For this review, take the finished solid that the model builds, in its own axes (mm). Coordinates: 2 decimals unless noted, no trailing zeros. Loops run counter-clockwise (first coordinate to the right, second up) from the corner with the lowest first, then second, coordinate; pieces in that order, holes last. Notation, with made-up numbers: M 6,50 L 64,50 A25 cw 64,77 Z; hole C 59,12 d5. An arc over 180 degrees is marked long. Put each result on its own line as item: value.
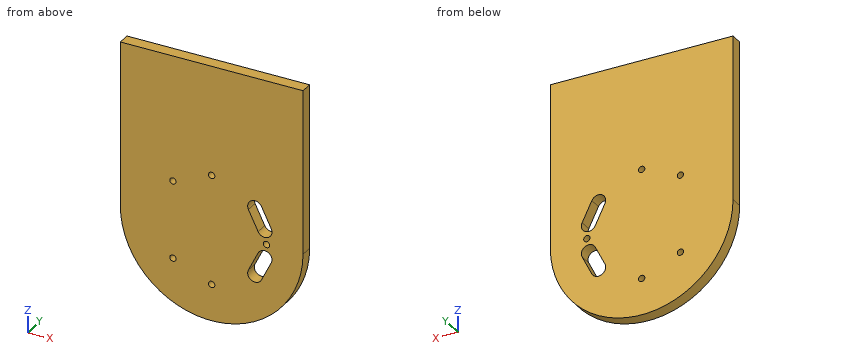
```python
from build123d import *

# Parameters (mm, degrees)
SKETCH1_R           = 47.625
SKETCH1_R_2         = 1.651
BOSS_EXTRUDE1_DEPTH = 6.35


with BuildPart() as part:
    # Sketch1 → Boss-Extrude1 (new body)
    # profile 1 of 3: a face of its own
    with BuildSketch(Plane(origin=(0, 0, 0), x_dir=(1, 0, 0), z_dir=(0, 1, 0))):
        Circle(SKETCH1_R)
        with Locations(Location((0, 28.575, 0), (0, 0, 270))):
            Circle(SKETCH1_R_2, mode=Mode.SUBTRACT)
        with Locations(Location((0, -28.575, 0), (0, 0, 270))):
            Circle(SKETCH1_R_2, mode=Mode.SUBTRACT)
        with Locations(Location((28.575, 0, 0), (0, 0, 270))):
            Circle(SKETCH1_R_2, mode=Mode.SUBTRACT)
        with Locations(Location((-20.205576272, 20.205576272, 0), (0, 0, 270))):
            Circle(SKETCH1_R_2, mode=Mode.SUBTRACT)
        with Locations(Location((-20.205576272, -20.205576272, 0), (0, 0, 270))):
            Circle(SKETCH1_R_2, mode=Mode.SUBTRACT)
        with BuildLine():
            ThreePointArc((25.985410077, 19.213209427), (20.881913097, 20.941364101), (19.153758423, 15.837867121))
            Line((19.153758423, 15.837867121), (24.216771881, 5.59038964))
            ThreePointArc((24.216771881, 5.59038964), (29.320268861, 3.862234966), (31.048423535, 8.965731946))
            Line((31.048423535, 8.965731946), (25.985410077, 19.213209427))
        make_face(mode=Mode.SUBTRACT)
        with BuildLine():
            Line((31.048423535, -8.965731946), (25.985410077, -19.213209427))
            ThreePointArc((25.985410077, -19.213209427), (20.881913097, -20.941364101), (19.153758423, -15.837867121))
            Line((19.153758423, -15.837867121), (24.216771881, -5.59038964))
            ThreePointArc((24.216771881, -5.59038964), (29.320268861, -3.862234966), (31.048423535, -8.965731946))
        make_face(mode=Mode.SUBTRACT)
    # profile 2 of 3: a face of its own
    with BuildSketch(Plane(origin=(0, 0, 0), x_dir=(1, 0, 0), z_dir=(0, 1, 0))):
        with BuildLine():
            Line((0, -85.725), (0, -47.625))
            ThreePointArc((0, -47.625), (-33.675960454, -33.675960454), (-47.625, 0))
            Line((-47.625, 0), (-47.625, -85.725))
            Line((-47.625, -85.725), (0, -85.725))
        make_face()
    # profile 3 of 3: a face of its own
    with BuildSketch(Plane(origin=(0, 0, 0), x_dir=(1, 0, 0), z_dir=(0, 1, 0))):
        with BuildLine():
            ThreePointArc((47.625, 0), (33.675960454, -33.675960454), (0, -47.625))
            Line((0, -47.625), (0, -85.725))
            Line((0, -85.725), (47.625, -85.725))
            Line((47.625, -85.725), (47.625, 0))
        make_face()
    extrude(amount=BOSS_EXTRUDE1_DEPTH)


solid = part.part
```
(1) Add section C-C (x = -33). Write out the cut boundary in (y, z) (3 decimals), plus the area to 3 significant figures.
Determined:
outline: M 0,-34.339 L 6.35,-34.339 L 6.35,85.725 L 0,85.725 Z
area: 762 mm^2
(2) Add section B-B (y = 1). Write out the cut boundary in (x, z) (3 decimals), plus the area to 3 significant figures.
Determined:
outline: M -47.625,0 A47.625 ccw 47.625,0 L 47.625,85.725 L -47.625,85.725 Z; hole C -20.206,-20.206 d3.302; hole C -20.206,20.206 d3.302; hole C 0,-28.575 d3.302; hole C 0,28.575 d3.302; hole M 19.154,-15.838 A3.81 ccw 25.985,-19.213 L 31.048,-8.966 A3.81 ccw 24.217,-5.59 Z; hole M 19.154,15.838 L 24.217,5.59 A3.81 ccw 31.048,8.966 L 25.985,19.213 A3.81 ccw Z; hole C 28.575,0 d3.302
area: 11,400 mm^2
(3) For pin 1 (4.5 mm diameter, centred on x = -20.21, z = 20.21, fed in from -Y); pin 2 (2 mm diameter, centred on x = 0, z = -28.575, fed in from +Y), all flat-tipped, find the tip position at first contact; note any pin that passes through.
Determined:
pin 1: stops at y = 0
pin 2: passes through
(4) Wall thickness on line 1 along Z through (x, y) = (21, 4.25) (3 decimals); line 2 along X through (y, z) = (2.5, -17.5); line 3 along X through (y, z) = (5.75, -30): over which ranges is each line inside the solid? List them lowest first. Write a range as [from, to].
Determined:
line 1: z = [-42.745, -20.997], [-12.101, 12.101], [20.997, 85.725]
line 2: x = [-44.29, 18.76], [26.83, 44.29]
line 3: x = [-36.99, -0.83], [0.83, 36.99]
(5) Add section A-A (x = 0). Write out the cut boundary in (y, z) (3 decimals).
Determined:
outline: M 0,-47.625 L 6.35,-47.625 L 6.35,-30.226 L 0,-30.226 Z; M 0,-26.924 L 6.35,-26.924 L 6.35,26.924 L 0,26.924 Z; M 0,30.226 L 6.35,30.226 L 6.35,85.725 L 0,85.725 Z
